Geometry: final body of the model. Coordinates: model frame, mm. Face numbers are marked on the shaded views. A direction names the side the tool comes from. Round coordinates to 2 decimals unless told otherwise and drop trailing zeros. Loops run counter-clockwise (first coordinate to the right, second up) from the corner with the lowest first, then second, coordinate; pieces in that order, holes last. Notation, with made-up numbers: (51.5, 72) - (65.5, 72) arc R24 cw to (65.5, 85) - close; hole circle Ø1 at (74.25, 54.25). An arc over 180 degrees is marked (long way). Answer as a JSON object with one key per item and string values. Group by question number.
Item 1: Section B-B (z = 8.25). Return the cut outline in (x, y), plus the area to 3 significant figures.
Item 2: First-contact query: pin 1 (3 mm diameter, centred on y = 55, z = 14.5, fed in from +X); pin 2 (1 mm diameter, centred on y = 58, z = 3, fed in from -X); pin 3 (6 mm diameter, centred on x = -21.5, y = 60.5, fed in from -Z); pin 4 (8 mm diameter, centred on y = 51.5, z = 16, fed in from -X). Flat tips, straight axial feed; report the tip coordinate or a pass-through.
Item 3: Section D-D (y = 62.5). Return the cut outline in (x, z).
Item 4: Section C-C (x = -32.5). Return the cut outline in (y, z), plus the area to 3 significant figures.
Item 5: Section A-A (x = -22). Return the cut outline in (y, z).
Item 6: Line query: line 1 (Y direction, x = -29, z = 8); line 2 (Y direction, x = -22, z = 7.75); line 3 (X direction, y = 49.25, z = 16.75). Output: solid intervals per line, ascending.
Item 7: Draft query along Y for the marked faces 1, 2 and 3. Return one class per face: released by +Y, released by -Y, zero draft, split by the parting line, or undercut.
Item 8: Reachability of the marked faces 4 and 5 from +Z, -Z, +X, -X, +Y, -Y: full face, straight path, thin tool, end or side. Return the list, or none.
```python
from build123d import *

# Parameters (mm, degrees)
F1_DEPTH    = 18
F2_T1_DEPTH = 25.5
F2_T3_DEPTH = 20.8647450844


# Not quite as in the source:
# - a fillet or chamfer that OpenCascade refuses, or shapes differently, is made with other operations: its cross-section is extruded or revolved along the edge and cut away or added


with BuildPart() as f1:
    # F0 (on Top) → F1 (new body)
    with BuildSketch(Plane.XY):
        Polygon((-16.1896759786, 48.2207899958), (-34.8480351921, 48.2207899958), (-34.8480351921, 46.7207899958), (-14.8480351921, 46.7207899958), (-14.8480351921, 48.2207899958), (-31.5147018588, 66.8546898083), (-31.523009312, 65.3639778233), align=None)
    extrude(amount=F1_DEPTH)

    # F2: fillet of radius 1.5 on 3 edges, made by hand

    # F2_s2 → F2_t1 (cut)
    with BuildSketch(Plane.XY.offset(-3.75)):
        with BuildLine():
            ThreePointArc((-16.3480351921, 46.7207899958), (-15.2873750203, 47.160129824), (-14.8480351921, 48.2207899958))
            Line((-14.8480351921, 48.2207899958), (-14.8480351921, 46.7207899958))
            Line((-14.8480351921, 46.7207899958), (-16.3480351921, 46.7207899958))
        make_face()
        with BuildLine():
            ThreePointArc((-33.3480351921, 48.2207899958), (-34.4086953639, 47.7814501676), (-34.8480351921, 46.7207899958))
            Line((-34.8480351921, 46.7207899958), (-34.8480351921, 48.2207899958))
            Line((-34.8480351921, 48.2207899958), (-33.3480351921, 48.2207899958))
        make_face()
    extrude(amount=F2_T1_DEPTH, mode=Mode.SUBTRACT)

    # F2_s4 → F2_t3 (cut)
    with BuildSketch(Plane.XY.offset(-1.4323725422)):
        with BuildLine():
            ThreePointArc((-14.8480351921, 47.6478409789), (-14.9467766537, 48.1830741136), (-15.2300012034, 48.6478409789))
            Line((-15.2300012034, 48.6478409789), (-14.8480351921, 48.2207899958))
            Line((-14.8480351921, 48.2207899958), (-14.8480351921, 47.6478409789))
        make_face()
    extrude(amount=F2_T3_DEPTH, mode=Mode.SUBTRACT)


solid = f1.part
```
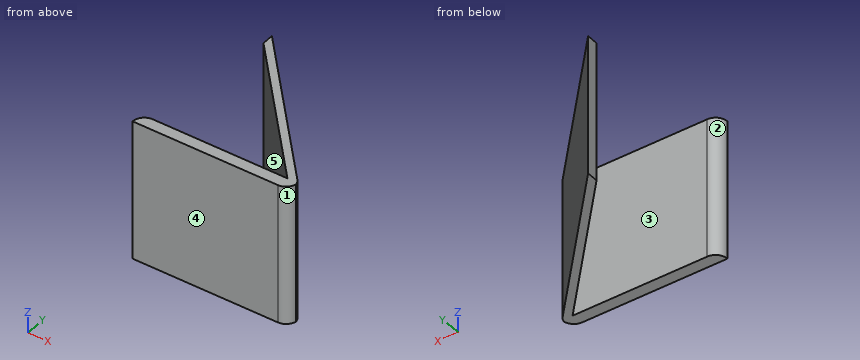
Values:
{
 "1": {"outline": "(-34.85, 46.72) - (-16.35, 46.72) arc R1.5 ccw to (-14.88, 47.93) arc R1.5 ccw to (-15.23, 48.65) - (-31.51, 66.85) - (-31.52, 65.36) - (-16.19, 48.22) - (-33.35, 48.22) arc R1.5 ccw to start", "area": "53.0 mm^2"},
 "2": {"pin 1": "stops at x = -19.57", "pin 2": "stops at x = -25.38", "pin 3": "passes through", "pin 4": "stops at x = -34.63"},
 "3": {"outline": "(-28.96, 0) - (-27.62, 0) - (-27.62, 18) - (-28.96, 18) - close"},
 "4": {"outline": "(46.72, 0) - (48.22, 0) - (48.22, 18) - (46.72, 18) - close", "area": "27.0 mm^2"},
 "5": {"outline": "(46.72, 0) - (48.22, 0) - (48.22, 18) - (46.72, 18) - close; (54.72, 0) - (56.22, 0) - (56.22, 18) - (54.72, 18) - close"},
 "6": {"line 1": "y = 46.72 to 48.22, 62.54 to 64.04", "line 2": "y = 46.72 to 48.22, 54.72 to 56.22", "line 3": "x = -17.11 to -15.77"},
 "7": {"face 1": "released by -Y", "face 2": "released by +Y", "face 3": "undercut"},
 "8": {"face 4": "+Z, -Z, +X, -X, -Y", "face 5": "+Z, -Z, -X"}
}
